Here's how the part is built. I have some questions about the finished solid (model axes, mm). Give positions to 0.01 mm unless a question says otherwise; leave off trailing zeros. Loops run counter-clockwise (first coordinate to the right, second up) from the corner with the lowest first, then second, coordinate; pieces in that order, holes last.
Q1. We'd pull the mould along X, two halves only. Please class faces 1 (the face through (-13.999, 4.19, -4.964)), 2 (the face through (-2, 4, 8)), 3 (the face through (-24.627, 4.19, -31.774)): +X half, -X half, draft (parallel to the pull), parting line (faces both ways), or undercut.
Q2. If we section it at C-C (y = 2): Please give me the cut outline in (x, z), plus the area to 3 significant figures.
Q3. Will these pins go through, and if not, where does the flat tip stop? P1, Ø1, axis at y = 6, z = 1.5, coming from the -X side; P2, Ø1.5, axis at y = 3.5, z = -8.5, coming from the +X side; P3, Ø1.8, axis at x = -12, z = -15, coming from the -Y side; P4, Ø5, axis at x = -8.5, y = 1.5, coming from the +Z side.
Q4. If we section it at B-B (x = -12): Please give me the cut outline in (y, z), plus the area to 3 significant figures.
Q5. If we section it at A-A (z = -15): Please give me the cut outline in (x, y).
Q6. If we section it at D-D (z = 4): Please give me the cut outline in (x, y), plus the area to 3 significant figures.
Q7. I need wall thicknesses on line 1 (X direction, y = 1.75, z = -16); line 2 (Z direction, x = -12, y = 2); line 3 (Z direction, x = -24.5, y = 1.5). Which ranges of each line are inside material? Lowest first, please.
from build123d import *

# Parameters (mm, degrees)
CROQUIS1_R              = 1.5
SALIENTE_EXTRUIR1_DEPTH = 8.5


with BuildPart() as part:
    # Croquis1 → Saliente-Extruir1 (new body)
    with BuildSketch(Plane(origin=(0, 0, 0), x_dir=(1, 0, 0), z_dir=(0, 1, 0))):
        with BuildLine():
            Line((-29.118820837, 29.661035883), (-16.013814133, 12.018507739))
            ThreePointArc((-16.013814133, 12.018507739), (-13.96004638, 4.867227057), (-10.5, -1.719642946))
            ThreePointArc((-10.5, -1.719642946), (-7.591888883, -5.213667237), (-4, -8))
            Line((-4, -8), (0, -8))
            Line((0, -8), (0, 4))
            ThreePointArc((0, 4), (-4.364647968, 5.683377936), (-6.468572218, 9.861585197))
            Line((-6.468572218, 9.861585197), (-7.024175217, 15.49108831))
            ThreePointArc((-7.024175217, 15.49108831), (-7.25881516, 16.587818098), (-7.732007274, 17.604657001))
            Line((-7.732007274, 17.604657001), (-19.180652605, 36.364414997))
            ThreePointArc((-19.180652605, 36.364414997), (-27.657401297, 38.213052032), (-29.118820837, 29.661035883))
        make_face()
        with Locations((-24.302243876, 33.238826596)):
            Circle(CROQUIS1_R, mode=Mode.SUBTRACT)
        with Locations((-12, 15)):
            Circle(CROQUIS1_R, mode=Mode.SUBTRACT)
    extrude(amount=SALIENTE_EXTRUIR1_DEPTH)


solid = part.part
Check sheet entries:
1. face 1: -X half
1. face 2: draft
1. face 3: undercut
2. outline: (-29.12, -29.66) arc R6 ccw (long way) to (-19.18, -36.36) - (-7.73, -17.6) arc R5 ccw to (-7.02, -15.49) - (-6.47, -9.86) arc R6.5 cw to (0, -4) - (0, 8) - (-4, 8) arc R21 ccw to (-10.5, 1.72) arc R36.53 ccw to (-16.01, -12.02) - close; hole circle Ø3 at (-24.3, -33.24); hole circle Ø3 at (-12, -15)
2. area: 509 mm2
3. P1: stops at x = -10.97
3. P2: stops at x = -5.89
3. P3: passes through
3. P4: stops at z = 6.6
4. outline: (0, -24.6) - (8.5, -24.6) - (8.5, -16.5) - (0, -16.5) - close; (0, -13.5) - (8.5, -13.5) - (8.5, -0.75) - (0, -0.75) - close
4. area: 177 mm2
5. outline: (-18.23, 0) - (-13.5, 0) - (-13.5, 8.5) - (-18.23, 8.5) - close; (-10.5, 0) - (-6.98, 0) - (-6.98, 8.5) - (-10.5, 8.5) - close
6. outline: (-8.75, 0) - (0, 0) - (0, 8.5) - (-8.75, 8.5) - close
6. area: 74.4 mm2
7. line 1: x = -18.97 to -13.12, -10.88 to -7.1
7. line 2: z = -24.6 to -16.5, -13.5 to -0.75
7. line 3: z = -39.24 to -34.73, -31.75 to -23.44
